Check sheet for the modelled part. Datum: model origin and axes. Units: mm. A direction names the side the tool comes from. Coordinates: 2 decimals unless noted, no trailing zeros. Order: outer loops, then holes, each group sorted by start corner. A loop starts at its lowest first (then second) coordinate and runs counter-clockwise, first axis right, second up.
1. Set-up check for faces 4 (the flat face through (0, -11.5, 102)), 5 (the flat face through (-21.5, 0, 120)), 6 (the flat face through (0, 13.7, 102)): record each of +Z, -Z, +X, -X, +Y, -Y from which the full face is reachable in a straight line by a thin tool's end or side.
2. Cross-section at C-C (x = 2). Enter the section's corners in (y, z).
3. Cross-section at B-B (y = -4). Enter the section's corners in (x, z), then the cut area to 3 significant figures.
4. Cross-section at A-A (z = 124). Enter the section's corners in (x, y).
5. Cross-section at D-D (z = 16). Count the separate pieces of the cut face and the enclosed holes in it, then the cut area to 3 significant figures.
6. Gauge pin test, flat ends, axial feed: pin 1 Ø0.7 at (y, z) = (-13, 103) entering from +X; pin 2 Ø4 at (x, y) = (-16.5, 0) entering from -Z; pin 3 Ø4 at (x, z) = (19.5, 110.5) entering from +Y; pin 4 Ø2.5 at (x, y) = (-18.5, 0.5) entering from +Z. Record the tip position at first contact, or that the pin passes through.
7. Thickness scan on line 1 (Z direction, x = -20, y = 3); line 2 (Y direction, x = -31.5, z = 15.5); line 3 (Y direction, x = -25, z = 45) (3 decimals). Record the ranges inside material, lowest first.
8. Draft check along Y on faces 1 (the flat face through (0, -13.7, 102)), 2 (the flat face through (-19, -1.1, 120)), 3 (the flat face through (35, -22, 0)). Enter one of: released by +Y, released by -Y, zero draft, split by the parting line, or undercut.
Autodesk Fusion 360 part; units mm, degrees
ref_plane "WorkPlane1" through (0, 0, 100) normal (0, 0, 1) x (1, 0, 0)
ref_plane "WorkPlane2" through (0, 0, 100) normal (0, 0, 1) x (1, 0, 0)
ref_plane "WorkPlane3" through (0, 0, 100) normal (0, 0, 1) x (1, 0, 0)
ref_plane "WorkPlane4" through (0, 0, 100) normal (0, 0, 1) x (1, 0, 0)
ref_plane "WorkPlane5" through (0, 0, 100) normal (0, 0, 1) x (1, 0, 0)
ref_plane "WorkPlane6" through (0, 0, 100) normal (0, 0, 1) x (1, 0, 0)
ref_plane "WorkPlane7" through (0, 0, 100) normal (0, 0, 1) x (1, 0, 0)
ref_plane "WorkPlane8" through (0, 0, 100) normal (0, 0, 1) x (1, 0, 0)
ref_plane "WorkPlane9" through (0, 0, 100) normal (0, 0, 1) x (1, 0, 0)
ref_plane "WorkPlane10" through (0, 0, 100) normal (0, 0, 1) x (1, 0, 0)
ref_plane "WorkPlane11" through (0, 0, 100) normal (0, 0, 1) x (1, 0, 0)
ref_plane "WorkPlane12" through (0, 0, 100) normal (0, 0, 1) x (1, 0, 0)
ref_plane "WorkPlane13" through (0, 0, 100) normal (0, 0, 1) x (1, 0, 0)
ref_plane "WorkPlane14" through (0, 0, 100) normal (0, 0, 1) x (1, 0, 0)
ref_plane "WorkPlane15" through (0, 0, 100) normal (0, 0, 1) x (1, 0, 0)
ref_plane "WorkPlane16" through (0, 0, 100) normal (0, 0, 1) x (1, 0, 0)
ref_plane "WorkPlane18" through (0, 0, 100) normal (0, 0, 1) x (1, 0, 0)
ref_plane "WorkPlane20" through (0, 0, 100) normal (0, 0, 1) x (1, 0, 0)
ref_plane "WorkPlane21" through (0, 0, 105) normal (0, 0, 1) x (1, 0, 0)
ref_plane "WorkPlane22" through (0, 0, 100) normal (0, 0, 1) x (1, 0, 0)
ref_plane "WorkPlane23" through (0, 0, 105) normal (0, 0, 1) x (1, 0, 0)
ref_plane "WorkPlane25" through (0, 0, 105) normal (0, 0, 1) x (1, 0, 0)
ref_plane "WorkPlane26" through (0, 0, 100) normal (0, 0, 1) x (1, 0, 0)
ref_plane "WorkPlane27" through (0, 0, 100) normal (0, 0, 1) x (1, 0, 0)
ref_plane "WorkPlane28" through (0, 0, 105) normal (0, 0, 1) x (1, 0, 0)
ref_plane "WorkPlane29" through (0, 0, 100) normal (0, 0, 1) x (1, 0, 0)
ref_plane "WorkPlane31" through (0, 0, 105) normal (0, 0, 1) x (1, 0, 0)
ref_plane "WorkPlane32" through (0, 0, 100) normal (0, 0, 1) x (1, 0, 0)
ref_plane "WorkPlane33" through (0, 0, 105) normal (0, 0, 1) x (1, 0, 0)
ref_plane "WorkPlane34" through (0, 0, 0) normal (0, 0, 1) x (1, 0, 0)
ref_plane "WorkPlane35" through (0, 0, 0) normal (0, 0, 1) x (1, 0, 0)
ref_plane "WorkPlane36" through (0, 0, 0) normal (0, 0, 1) x (1, 0, 0)
ref_plane "WorkPlane37" through (0, 0, 0) normal (0, 0, 1) x (1, 0, 0)
ref_plane "WorkPlane38" through (0, 0, 100) normal (0, 0, 1) x (1, 0, 0)
ref_plane "WorkPlane39" through (0, 0, 100) normal (0, 0, 1) x (1, 0, 0)
ref_plane "WorkPlane40" through (0, 0, 105) normal (0, 0, 1) x (1, 0, 0)
ref_plane "WorkPlane41" through (0, 0, 0) normal (0, 0, 1) x (1, 0, 0)
ref_plane "WorkPlane42" through (0, 0, 0) normal (0, 0, 1) x (1, 0, 0)
ref_plane "WorkPlane43" through (0, 0, 0) normal (0, 0, 1) x (1, 0, 0)
ref_plane "WorkPlane44" through (0, 0, 0) normal (0, 0, 1) x (1, 0, 0)
ref_plane "WorkPlane45" through (0, 0, 100) normal (0, 0, 1) x (1, 0, 0)
ref_plane "WorkPlane46" through (0, 0, 100) normal (0, 0, 1) x (1, 0, 0)
ref_plane "WorkPlane47" through (0, 0, 100) normal (0, 0, 1) x (1, 0, 0)
ref_plane "WorkPlane48" through (0, 0, 100) normal (0, 0, 1) x (1, 0, 0)
ref_plane "WorkPlane49" through (0, 0, 0) normal (0, 0, 1) x (1, 0, 0)
ref_plane "WorkPlane50" through (0, 0, 100) normal (0, 0, 1) x (1, 0, 0)
ref_plane "WorkPlane51" through (0, 0, 0) normal (0, 0, 1) x (1, 0, 0)
ref_plane "WorkPlane52" through (0, 0, 100) normal (0, 0, 1) x (1, 0, 0)
ref_plane "WorkPlane53" through (0, 0, 0) normal (0, 0, 1) x (1, 0, 0)
ref_plane "WorkPlane54" through (0, 0, 100) normal (0, 0, 1) x (1, 0, 0)
ref_plane "WorkPlane55" through (0, 0, 0) normal (0, 0, 1) x (1, 0, 0)
ref_plane "WorkPlane56" through (0, 0, 100) normal (0, 0, 1) x (1, 0, 0)
ref_plane "WorkPlane57" through (0, 0, 100) normal (0, 0, 1) x (1, 0, 0)
ref_plane "WorkPlane58" through (0, 0, 0) normal (0, 0, 1) x (1, 0, 0)
ref_plane "WorkPlane59" through (0, 0, 100) normal (0, 0, 1) x (1, 0, 0)
sketch "Sketch240" plane through (0, 0, 0) normal (0, 0, 1) x (1, 0, 0)
  line L0 (31, 18) -> (39, 18)
  line L1 (39, 18) -> (39, 26)
  line L2 (39, 26) -> (31, 26)
  line L3 (31, 26) -> (31, 18)
sketch "Sketch241" plane through (0, 0, 100) normal (0, 0, 1) x (1, 0, 0)
  line L0 (11.7, 5.7) -> (19.7, 5.7)
  line L1 (19.7, 5.7) -> (19.7, 13.7)
  line L2 (19.7, 13.7) -> (11.7, 13.7)
  line L3 (11.7, 13.7) -> (11.7, 5.7)
loft "Loft97" add profiles "Sketch240", "Sketch241" section 1 section 2 makes body 1
ref_plane "WorkPlane60" through (0, 0, 0) normal (0, 0, 1) x (1, 0, 0)
ref_plane "WorkPlane61" through (0, 0, 100) normal (0, 0, 1) x (1, 0, 0)
sketch "Sketch242" plane through (0, 0, 0) normal (0, 0, 1) x (1, 0, 0)
  line L0 (-39, 18) -> (-31, 18)
  line L1 (-31, 18) -> (-31, 26)
  line L2 (-31, 26) -> (-39, 26)
  line L3 (-39, 26) -> (-39, 18)
sketch "Sketch243" plane through (0, 0, 100) normal (0, 0, 1) x (1, 0, 0)
  line L0 (-19.7, 5.7) -> (-11.7, 5.7)
  line L1 (-11.7, 5.7) -> (-11.7, 13.7)
  line L2 (-11.7, 13.7) -> (-19.7, 13.7)
  line L3 (-19.7, 13.7) -> (-19.7, 5.7)
loft "Loft98" add profiles "Sketch242", "Sketch243" section 1 section 2 separate body makes body 2
ref_plane "WorkPlane62" through (0, 0, 0) normal (0, 0, 1) x (1, 0, 0)
ref_plane "WorkPlane63" through (0, 0, 100) normal (0, 0, 1) x (1, 0, 0)
sketch "Sketch244" plane through (0, 0, 0) normal (0, 0, 1) x (1, 0, 0)
  line L0 (-39, -26) -> (-31, -26)
  line L1 (-31, -26) -> (-31, -18)
  line L2 (-31, -18) -> (-39, -18)
  line L3 (-39, -18) -> (-39, -26)
sketch "Sketch245" plane through (0, 0, 100) normal (0, 0, 1) x (1, 0, 0)
  line L0 (-19.7, -13.7) -> (-11.7, -13.7)
  line L1 (-11.7, -13.7) -> (-11.7, -5.7)
  line L2 (-11.7, -5.7) -> (-19.7, -5.7)
  line L3 (-19.7, -5.7) -> (-19.7, -13.7)
loft "Loft99" add profiles "Sketch244", "Sketch245" section 1 section 2 separate body makes body 3
ref_plane "WorkPlane64" through (0, 0, 0) normal (0, 0, 1) x (1, 0, 0)
ref_plane "WorkPlane65" through (0, 0, 100) normal (0, 0, 1) x (1, 0, 0)
sketch "Sketch246" plane through (0, 0, 0) normal (0, 0, 1) x (1, 0, 0)
  line L0 (31, -26) -> (39, -26)
  line L1 (39, -26) -> (39, -18)
  line L2 (39, -18) -> (31, -18)
  line L3 (31, -18) -> (31, -26)
sketch "Sketch247" plane through (0, 0, 100) normal (0, 0, 1) x (1, 0, 0)
  line L0 (11.7, -13.7) -> (19.7, -13.7)
  line L1 (19.7, -13.7) -> (19.7, -5.7)
  line L2 (19.7, -5.7) -> (11.7, -5.7)
  line L3 (11.7, -5.7) -> (11.7, -13.7)
loft "Loft100" add profiles "Sketch246", "Sketch247" section 1 section 2 separate body makes body 4
ref_plane "WorkPlane66" through (0, 0, 100) normal (0, 0, 1) x (1, 0, 0)
sketch "Sketch248" plane through (0, 0, 100) normal (0, 0, 1) x (1, 0, 0)
  line L0 (-19.7, -13.7) -> (19.7, -13.7)
  line L1 (19.7, -13.7) -> (19.7, 13.7)
  line L2 (19.7, 13.7) -> (-19.7, 13.7)
  line L3 (-19.7, 13.7) -> (-19.7, -13.7)
  line L4 (-17.5, -11.5) -> (17.5, -11.5)
  line L5 (17.5, -11.5) -> (17.5, 11.5)
  line L6 (17.5, 11.5) -> (-17.5, 11.5)
  line L7 (-17.5, 11.5) -> (-17.5, -11.5)
extrude "Extrude50" add sketch "Sketch248" along normal blind 5 bodies 1 2 3 4
ref_plane "WorkPlane67" through (0, 0, 105.1) normal (0, 0, 1) x (1, 0, 0)
sketch "sk_CutInner" plane through (0, 0, 105.1) normal (0, 0, 1) x (1, 0, 0)
  line L0 (-17.4, -11.4) -> (17.4, -11.4)
  line L1 (17.4, -11.4) -> (17.4, 11.4)
  line L2 (17.4, 11.4) -> (-17.4, 11.4)
  line L3 (-17.4, 11.4) -> (-17.4, -11.4)
extrude "Extrude51" cut sketch "sk_CutInner" against normal blind 5.7 bodies 1
sketch "sk_RailRight" plane through (0, 0, 0) normal (0, 0, 1) x (1, 0, 0)
  line L0 (17.5, -11.5) -> (21.5, -11.5)
  line L1 (21.5, -11.5) -> (21.5, 11.5)
  line L2 (21.5, 11.5) -> (17.5, 11.5)
  line L3 (17.5, 11.5) -> (17.5, -11.5)
extrude "Extrude52" add sketch "sk_RailRight" along normal blind 140 separate body makes body 5
sketch "sk_GrooveRight" plane through (0, 0, 0) normal (0, 0, 1) x (1, 0, 0)
  line L0 (17.5, -1.1) -> (21, -1.1)
  line L1 (21, -1.1) -> (21, 1.1)
  line L2 (21, 1.1) -> (17.5, 1.1)
  line L3 (17.5, 1.1) -> (17.5, -1.1)
extrude "Extrude53" cut sketch "sk_GrooveRight" along normal blind 140 bodies 5
sketch "sk_TrimRailRight" plane through (0, 0, 0) normal (0, 0, 1) x (1, 0, 0)
  line L0 (17.5, -11.5) -> (21.5, -11.5)
  line L1 (21.5, -11.5) -> (21.5, 11.5)
  line L2 (21.5, 11.5) -> (17.5, 11.5)
  line L3 (17.5, 11.5) -> (17.5, -11.5)
extrude "Extrude54" cut sketch "sk_TrimRailRight" along normal blind 100 bodies 5
sketch "sk_RailLeft" plane through (0, 0, 0) normal (0, 0, 1) x (1, 0, 0)
  line L0 (-21.5, -11.5) -> (-17.5, -11.5)
  line L1 (-17.5, -11.5) -> (-17.5, 11.5)
  line L2 (-17.5, 11.5) -> (-21.5, 11.5)
  line L3 (-21.5, 11.5) -> (-21.5, -11.5)
extrude "Extrude55" add sketch "sk_RailLeft" along normal blind 140 separate body makes body 6
sketch "sk_GrooveLeft" plane through (0, 0, 0) normal (0, 0, 1) x (1, 0, 0)
  line L0 (-21, -1.1) -> (-17.5, -1.1)
  line L1 (-17.5, -1.1) -> (-17.5, 1.1)
  line L2 (-17.5, 1.1) -> (-21, 1.1)
  line L3 (-21, 1.1) -> (-21, -1.1)
extrude "Extrude56" cut sketch "sk_GrooveLeft" along normal blind 140 bodies 6
sketch "sk_TrimRailLeft" plane through (0, 0, 0) normal (0, 0, 1) x (1, 0, 0)
  line L0 (-21.5, -11.5) -> (-17.5, -11.5)
  line L1 (-17.5, -11.5) -> (-17.5, 11.5)
  line L2 (-17.5, 11.5) -> (-21.5, 11.5)
  line L3 (-21.5, 11.5) -> (-21.5, -11.5)
extrude "Extrude57" cut sketch "sk_TrimRailLeft" along normal blind 100 bodies 6
sketch "sk_BottomStop" plane through (0, 0, 0) normal (0, 0, 1) x (1, 0, 0)
  line L0 (-17.5, -1.2) -> (17.5, -1.2)
  line L1 (17.5, -1.2) -> (17.5, 1.2)
  line L2 (17.5, 1.2) -> (-17.5, 1.2)
  line L3 (-17.5, 1.2) -> (-17.5, -1.2)
extrude "Extrude58" add sketch "sk_BottomStop" along normal blind 103 separate body makes body 7
sketch "sk_TrimStop" plane through (0, 0, 0) normal (0, 0, 1) x (1, 0, 0)
  line L0 (-17.5, -1.2) -> (17.5, -1.2)
  line L1 (17.5, -1.2) -> (17.5, 1.2)
  line L2 (17.5, 1.2) -> (-17.5, 1.2)
  line L3 (-17.5, 1.2) -> (-17.5, -1.2)
extrude "Extrude59" cut sketch "sk_TrimStop" along normal blind 100 bodies 7
combine "Combine1" operation add target body 1 tool bodies 5 6 7
Data:
1. face 4: +Z
1. face 5: +Z, -X, +Y, -Y
1. face 6: +Z, +X, -X, +Y
2. outline: (-13.7, 100) - (-11.5, 100) - (-11.5, 105) - (-13.7, 105) - close; (-1.2, 100) - (1.2, 100) - (1.2, 103) - (-1.2, 103) - close; (11.5, 100) - (13.7, 100) - (13.7, 105) - (11.5, 105) - close
3. outline: (-21.5, 100) - (-17.5, 100) - (-17.5, 140) - (-21.5, 140) - close; (17.5, 100) - (21.5, 100) - (21.5, 140) - (17.5, 140) - close
3. area: 320 mm2
4. outline: (-21.5, -11.5) - (-17.5, -11.5) - (-17.5, -1.1) - (-21, -1.1) - (-21, 1.1) - (-17.5, 1.1) - (-17.5, 11.5) - (-21.5, 11.5) - close; (17.5, -11.5) - (21.5, -11.5) - (21.5, 11.5) - (17.5, 11.5) - (17.5, 1.1) - (21, 1.1) - (21, -1.1) - (17.5, -1.1) - close
5. separate pieces: 4
5. enclosed holes: 0
5. area: 256 mm2
6. pin 1: stops at x = 19.7
6. pin 2: stops at z = 100
6. pin 3: stops at y = 11.5
6. pin 4: stops at z = 140
7. line 1: z = 100 to 140
7. line 2: y = -24.09 to -16.09, 16.09 to 24.09
7. line 3: y = -20.465 to -12.465, 12.465 to 20.465
8. face 1: released by -Y
8. face 2: undercut
8. face 3: zero draft
